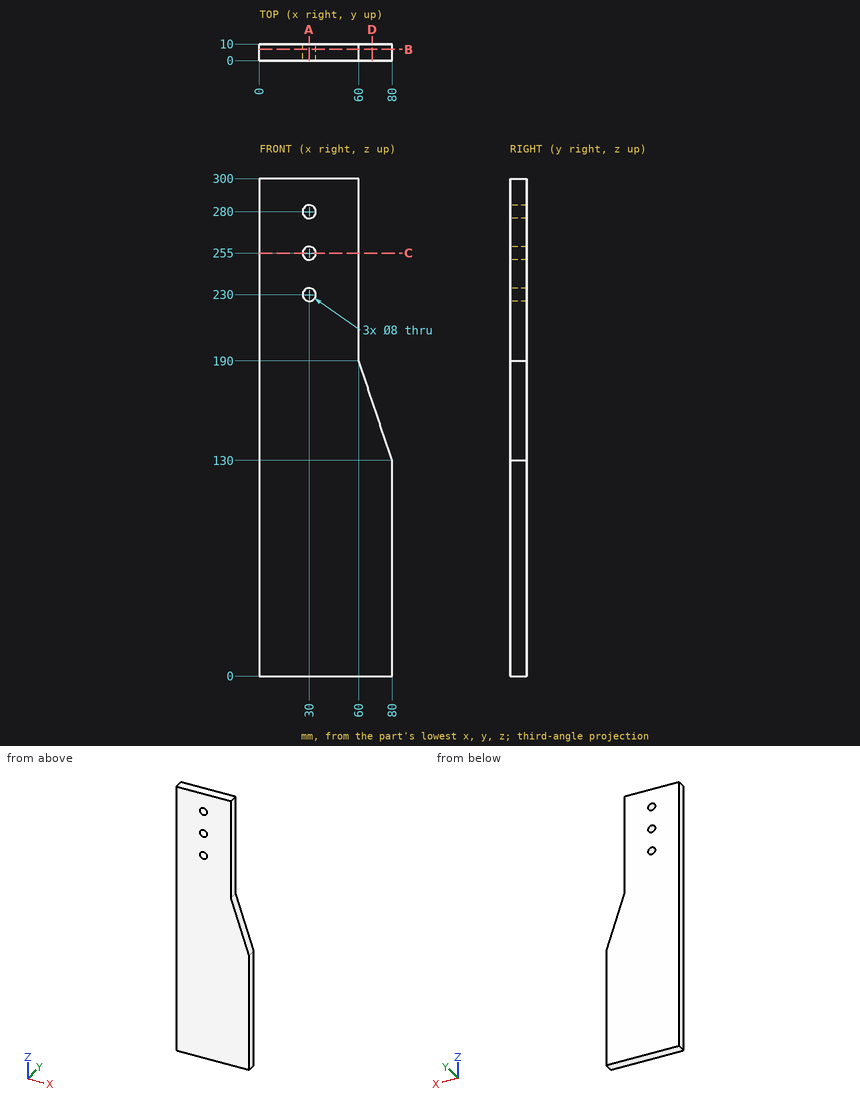
Can you work these out from the drawing? Everything is in mm from the part's minimum corner. Round coordinates to 2 decimals unless told otherwise and drop trailing zeros. Write each loop counter-clockwise with the first axis right and the second up, starting at its lowest first coordinate (ties: lowest second). Pieces come first, ordered by that corner, then holes. Notation, with made-up numbers: (8.25, 29.5) - (53.25, 29.5) arc R29 ccw to (53.25, 50.5) - close; hole circle Ø4 at (86, -30). An arc over 180 degrees is marked (long way). Write each question's results on one line, items separated by ' | '. Start each with the question number.
1) Suppose I cut it at B-B (y = 6.75). List the corners of the cut face in (x, z) for me, and give its area (3 significant figures).
2) Please list where these lines run through material, in increasing order: line 1 (Z direction, x = 30, y = 7); line 2 (X direction, y = 2.75, z = 280); line 3 (Z direction, x = 27, y = 1).
3) Suppose I cut it at C-C (z = 255). List the corners of the cut face in (x, y) for me.
4) Suppose I cut it at D-D (x = 68). List the corners of the cut face in (y, z) for me, and give its area (3 significant figures).
5) For pin 1 Ø9 at (x, z) = (30, 230) entering from +Y; pin 2 Ø5 at (y, z) = (7.5, 269.5) entering from +X; pin 3 Ø6 at (y, z) = (3.5, 145) entering from +X; pin 4 Ø5 at (x, z) = (30, 280) entering from -Y, each with a flat end and sliding along its axis, tell me the tip position at first contact or that it passes through.
6) Suppose I cut it at A-A (x = 30). List the corners of the cut face in (y, z) for me.
Here are the results:
1) outline: (0, 0) - (80, 0) - (80, 130) - (60, 190) - (60, 300) - (0, 300) - close; hole circle Ø8 at (30, 230); hole circle Ø8 at (30, 255); hole circle Ø8 at (30, 280) | area: 21,000 mm2
2) line 1: z = 0 to 226, 234 to 251, 259 to 276, 284 to 300 | line 2: x = 0 to 26, 34 to 60 | line 3: z = 0 to 227.35, 232.65 to 252.35, 257.65 to 277.35, 282.65 to 300
3) outline: (0, 0) - (26, 0) - (26, 10) - (0, 10) - close; (34, 0) - (60, 0) - (60, 10) - (34, 10) - close
4) outline: (0, 0) - (10, 0) - (10, 166) - (0, 166) - close | area: 1,660 mm2
5) pin 1: stops at y = 10 | pin 2: stops at x = 60 | pin 3: stops at x = 76 | pin 4: passes through
6) outline: (0, 0) - (10, 0) - (10, 226) - (0, 226) - close; (0, 234) - (10, 234) - (10, 251) - (0, 251) - close; (0, 259) - (10, 259) - (10, 276) - (0, 276) - close; (0, 284) - (10, 284) - (10, 300) - (0, 300) - close
